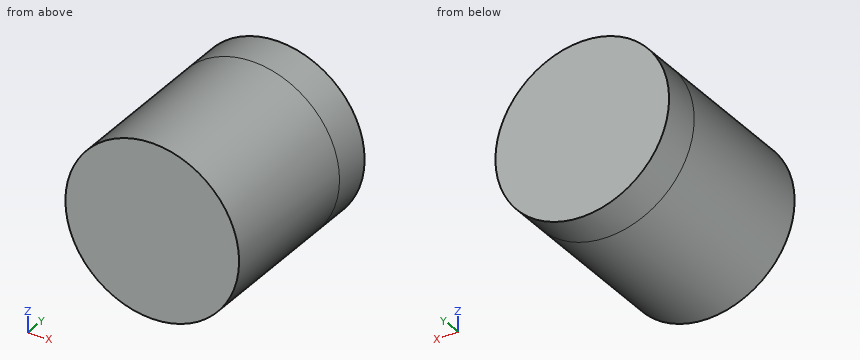
from build123d import *

# Parameters (mm, degrees)
F0_R     = 57.747245906
F1_DEPTH = 25.4
F2_DEPTH = 25.4
F3_DEPTH = 25.4
F4_DEPTH = 25.4
F7_DEPTH = 25.4


# Not quite as in the source:
# - the program builds the solid bodies; features that only make, move or delete a surface that nothing else refers to are left out


with BuildPart() as f1:
    # F0 (on Front) → F1 (new body)
    with BuildSketch(Plane.XZ):
        Circle(F0_R)
    extrude(amount=F1_DEPTH)

    # F2 (add): a face of the model
    f2_faces = [f1.faces().sort_by_distance(p)[0] for p in [
        (0, 0, 0),
    ]]
    extrude(f2_faces, amount=F2_DEPTH)

    # F3 (add): a face of the model
    f3_faces = [f1.faces().sort_by_distance(p)[0] for p in [
        (0, -25.4, 0),
    ]]
    extrude(f3_faces, amount=F3_DEPTH)

    # F4 (add): a face of the model
    f4_faces = [f1.faces().sort_by_distance(p)[0] for p in [
        (0, -50.8, 0),
    ]]
    extrude(f4_faces, amount=F4_DEPTH)

    # F7 (add): a face of the model
    f7_faces = [f1.faces().sort_by_distance(p)[0] for p in [
        (0, 25.4, 0),
    ]]
    extrude(f7_faces, amount=F7_DEPTH)


solid = f1.part
Design review of the part built by this model. Coordinates are the model's own, in mm. Coordinates: 2 decimals unless noted, no trailing zeros. Order: outer loops, then holes, each group sorted by start corner. A loop starts at its lowest first (then second) coordinate and runs counter-clockwise, first axis right, second up. Notation, with made-up numbers: (4.5, 69.25) -> (51.5, 69.25) arc R28 ccw to (51.5, 94.25) -> close; hole circle Ø5 at (27.5, -24.5). An arc over 180 degrees is marked (long way). Use one line per item in the form item = value. Start each with the question number.
(1) Add section A-A on y = -6.5. State the section outline as (x, z) points, plus the area to 3 significant figures.
(2) Add section B-B on z = -21. State the section outline as (x, y) points, plus the area to 3 significant figures.
(3) Insertion check: pin 1 (12 mm diameter, centred on y = -31, z = -14.5, fed in from +X); pin 2 (4 mm diameter, centred on x = -36.5, y = 27.5, fed in from +Z); pin 3 (4 mm diameter, centred on y = -42.5, z = -25, fed in from +X). Each pin has a flat end and moves straight along its axis. Give the tip position at first contact, or say it passes through.
(4) For probe 1 along Z at (x, y) = (1.5, -34); probe 2 along X at (y, z) = (-9.5, -1); probe 3 along Z at (x, y) = (7.5, 10), list the stretches that pass through material, from the lowest coordinate up.
(5) Add section C-C on x = 36. State the section outline as (y, z) points, plus the area to 3 significant figures.
Answer block:
q1.outline = circle Ø115.49 at (0, 0)
q1.area = 10,500 mm²
q2.outline = (-53.79, -76.2) -> (53.79, -76.2) -> (53.79, 50.8) -> (-53.79, 50.8) -> close
q2.area = 13,700 mm²
q3.pin_1 = 57.12
q3.pin_2 = 46.31
q3.pin_3 = 52.97
q4.probe_1 = -57.73 to 57.73
q4.probe_2 = -57.74 to 57.74
q4.probe_3 = -57.26 to 57.26
q5.outline = (-76.2, -45.15) -> (50.8, -45.15) -> (50.8, 45.15) -> (-76.2, 45.15) -> close
q5.area = 11,500 mm²
